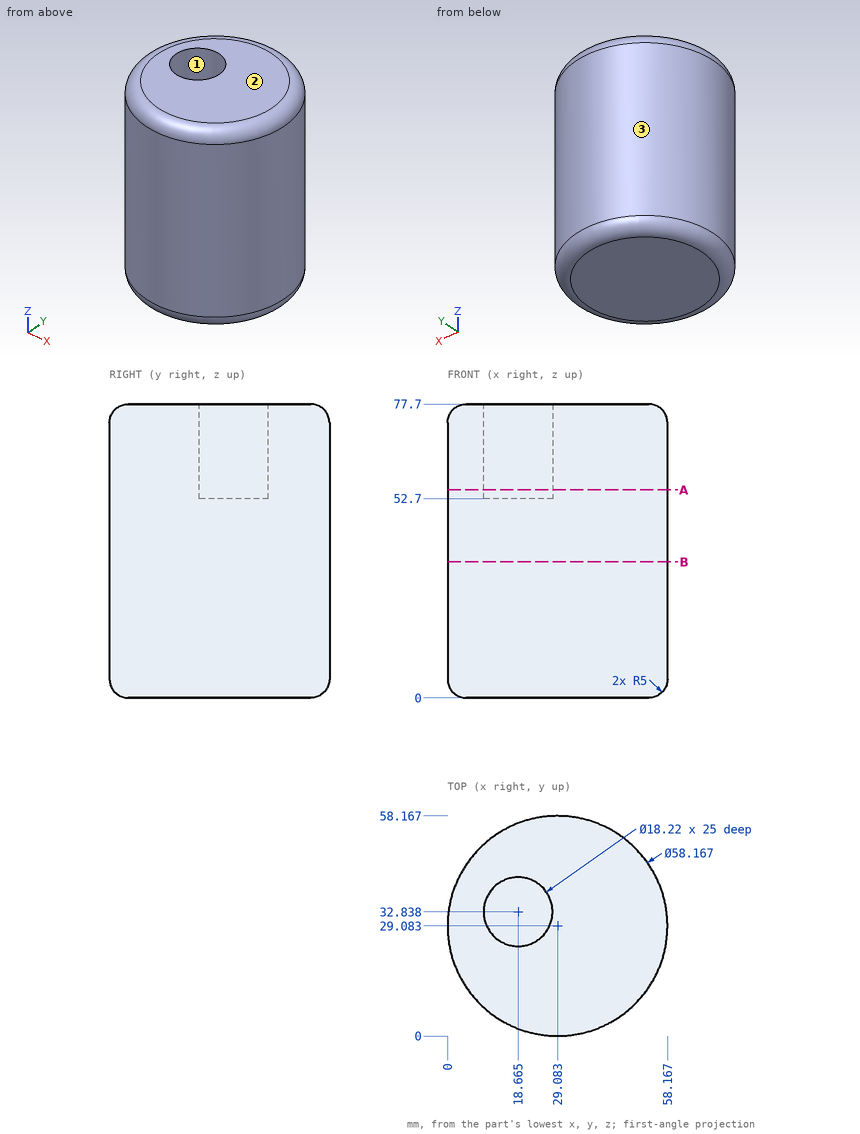
Study the drawing (mm; zero at the part's minimum x, y, z) and answer. Coordinates: 2 decimals unless noted, no trailing zeros. Write each loop counter-clockwise with the first axis right and the second up, starting at its lowest first coordinate (ties: lowest second). Pieces come first, ordered by that corner, then holes.
Q1. A cutting plane is placed at A-A, the plane z = 55. Give the vertices of the cut face in (x, y) (1 decimal).
Q2. Each of these flat-tipped pins is pushed along its axis until it touches: pin 1 Ø6 at (y, z) = (12, 52.5) entering from -X; pin 2 Ø1.5 at (y, z) = (6.5, 17.5) entering from -X; pin 3 Ø8 at (y, z) = (50.5, 47.5) entering from +X (1 decimal). Where does it stop, or does it pass through?
Q3. Determine the mould class of the marked faces 1, 2 and 3 for opening direction Y: released by +Y, released by -Y, zero draft, split by the parting line, or undercut.
Q4. A cutting plane is placed at B-B, the plane z = 36. Give the vertices of the cut face in (x, y), then the cut area to 3 significant figures.
Q5. Find the intervals of material crossed by line 1 (X direction, y = 28, z = 62.5) (1 decimal); line 2 (X direction, y = 29.5, z = 13); line 3 (Z direction, x = 23, y = 36), in increasing order.
Findings below:
1. outline: circle Ø58.2 at (29.1, 29.1); hole circle Ø18.2 at (18.7, 32.8)
2. pin 1: stops at x = 3.64
2. pin 2: stops at x = 9.87
2. pin 3: stops at x = 52.4
3. face 1: undercut
3. face 2: zero draft
3. face 3: split by the parting line
4. outline: circle Ø58.17 at (29.08, 29.08)
4. area: 2,660 mm2
5. line 1: x = 0 to 10.9, 26.4 to 58.1
5. line 2: x = 0 to 58.16
5. line 3: z = 0 to 52.7
